Part print with two shaded views. Sizes in mm from the minimum x, y, z corner. Round coordinates to 2 decimals unless told otherwise and drop trailing zeros. Loops run counter-clockwise (first coordinate to the right, second up) from the corner with the lowest first, then second, coordinate; pieces in that order, holes last.
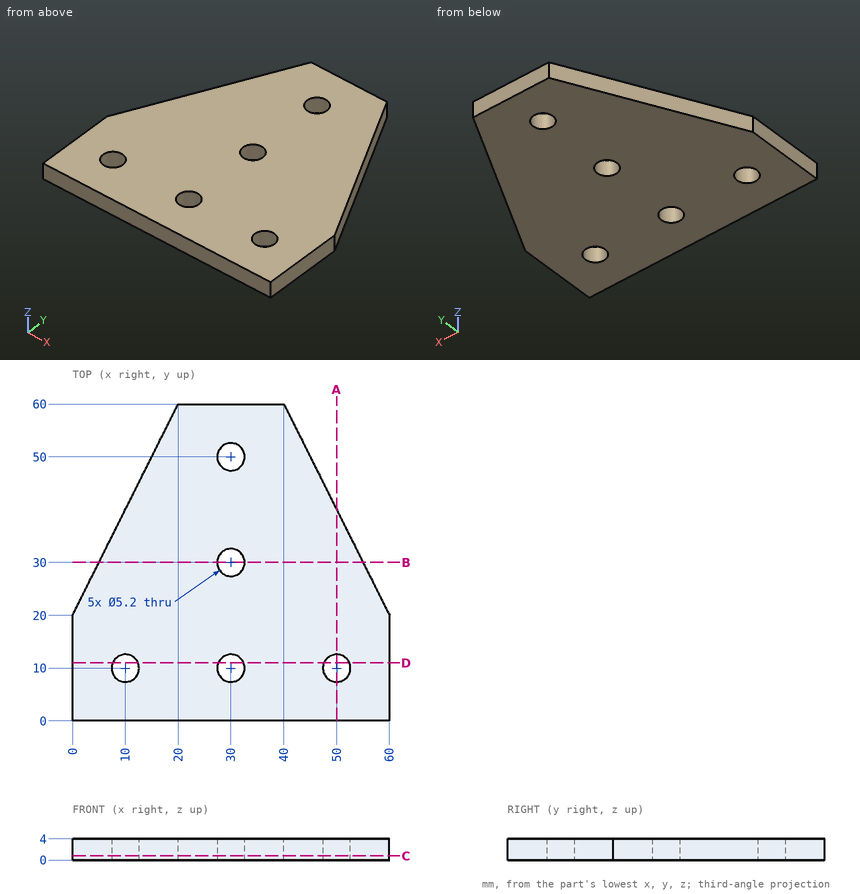
Item 1: Wall check: L1, parallel to Y at x = 30, z = 2.05; L2, parallel to Y at x = 50, z = 1.35; L3, parallel to X at y = 11, z = 2.05. Give the ranges that are in metal, low to high.
Verdict:
L1: y = 0 to 7.4, 12.6 to 27.4, 32.6 to 47.4, 52.6 to 60
L2: y = 0 to 7.4, 12.6 to 40
L3: x = 0 to 7.6, 12.4 to 27.6, 32.4 to 47.6, 52.4 to 60
Item 2: Cut at A-A (x = 50). List the corners of the cut face in (y, z).
Verdict:
outline: (0, 0) - (7.4, 0) - (7.4, 4) - (0, 4) - close; (12.6, 0) - (40, 0) - (40, 4) - (12.6, 4) - close
Item 3: Cut at D-D (y = 11). List the corners of the cut face in (x, z).
Verdict:
outline: (0, 0) - (7.6, 0) - (7.6, 4) - (0, 4) - close; (12.4, 0) - (27.6, 0) - (27.6, 4) - (12.4, 4) - close; (32.4, 0) - (47.6, 0) - (47.6, 4) - (32.4, 4) - close; (52.4, 0) - (60, 0) - (60, 4) - (52.4, 4) - close
Item 4: Cut at C-C (z = 0.8). List the corners of the cut face in (x, y).
Verdict:
outline: (0, 0) - (60, 0) - (60, 20) - (40, 60) - (20, 60) - (0, 20) - close; hole circle Ø5.2 at (10, 10); hole circle Ø5.2 at (30, 10); hole circle Ø5.2 at (30, 30); hole circle Ø5.2 at (30, 50); hole circle Ø5.2 at (50, 10)
Item 5: Cut at B-B (y = 30). List the corners of the cut face in (x, z).
Verdict:
outline: (5, 0) - (27.4, 0) - (27.4, 4) - (5, 4) - close; (32.6, 0) - (55, 0) - (55, 4) - (32.6, 4) - close
Item 6: Flat gauge pins, fed straight in: P1, Ø1, axis at x = 49.5, z = 1, coming from the +Y side; P2, Ø1, axis at x = 30.5, y = 48.5, coming from the -Z side. Where does each tip first touch, or does it go through?
Verdict:
P1: stops at y = 42
P2: passes through
